from build123d import *

# Parameters (mm, degrees)
PAD043_DEPTH        = 12.5
PAD044_DEPTH        = 57
PAD046_DEPTH        = 15
CUT_PLACEMENT_ANGLE = 180


with BuildPart() as body024:
    # Sketch100 → Pad043 (new body, symmetric)
    with BuildSketch(Plane.YZ):
        Polygon((43.43318, 10), (54.734671, 10), (60, 0), (48.698509, 0), align=None)
    extrude(amount=PAD043_DEPTH, both=True)


with BuildPart() as body024_1:
    # Body024 placement: moved
    add(body024.part.moved(Location((28.5, 0, 0))))


with BuildPart() as cut:
    # Sketch099 → Pad044 (new body)
    with BuildSketch(Plane.YZ):
        Polygon((0, 0), (60, 0), (54.734671, 10), (0, 10), align=None)
    extrude(amount=PAD044_DEPTH)

    # Sketch103 (on Face1 of Pad044) → Pad046 (join)
    with BuildSketch(Plane(origin=(0, 0, 10), x_dir=(0, -1, 0), z_dir=(0, 0, 1))):
        Polygon((0, 0), (-13.5, 0), (-13.5, 5), (-5, 5), (-5, 13.5), (0, 13.5), align=None)
        Polygon((0, 57), (-13.5, 57), (-13.5, 52), (-5, 52), (-5, 43.5), (0, 43.5), align=None)
    extrude(amount=PAD046_DEPTH)

    # Cut: cut Body024
    add(body024_1.part, mode=Mode.SUBTRACT)


with BuildPart() as cut_1:
    # Cut placement: moved
    add(cut.part.moved(Location((0, 5, 0))).rotate(Axis((0, 5, 0), (0, 1, 0)), CUT_PLACEMENT_ANGLE))


solid = cut_1.part
Geometry: final body of the model. Coordinates: model frame, mm. A direction names the side the tool comes from. Round coordinates to 2 decimals unless told otherwise and drop trailing zeros. Loops run counter-clockwise (first coordinate to the right, second up) from the corner with the lowest first, then second, coordinate; pieces in that order, holes last. Notation, with made-up numbers: M 67.25,83 L 116.25,83 A20 cw 116.25,96 Z; hole C 20.25,58.25 d1. An arc over 180 degrees is marked long. Put each result on its own line as item: value. Start each with the question number.
(1) Section query D-D (y = 12). Return loops of the section in (x, z), then the cut area to 3 significant figures.
(2) Set-up query: faces 1 (the face through (-2, 18.5, -17)), 2 (the face through (-43.5, 8, -17)), 3 (the face through (-4, 10, -25)), 4 (the face through (-9, 10, -17)). Return all of +Z, -Z, +X, -X, +Y, -Y with unobstructed straight access to the full face (end or side cutting, diameter ignored); none if empty.
(3) Section query B-B (z = -13). Return loops of the section in (x, y).
(4) Material intervals for line 1 along X through (y, z) = (53.5, -9.5); line 2 along X through (y, z) = (8.5, -20.25); line 3 along Z through (x, y) = (-35, 11), sorted ascending. Write a range as [from, to].
(5) Contact query for flat-ended pins moving along their axis: pin 1 Ø4 at (x, z) = (-48.5, -20) entering from +Y; pin 2 Ø3 at (x, y) = (-39.5, 37) entering from -Z; pin 3 Ø5.5 at (x, z) = (-2, -19.5) entering from +Y. Output: stop coordinate, or through.
(6) Section query A-A (y = 57). Return loops of the section in (x, z).
(7) Draft query along X for faces 5 (the face through (-57, 28, -7)), 6 (the face through (-16, 57, -5)), 7 (the face through (-55, 18.5, -17)). Return one class per face: +X half, -X half, draft (parallel to the pull), parting line (faces both ways), or undercut.
(8) Section query C-C (x = -48). Return loops of the section in (y, z), then the cut area to 3 significant figures.
Findings below:
1. outline: M -57,-25 L -52,-25 L -52,-10 L -5,-10 L -5,-25 L 0,-25 L 0,0 L -57,0 Z
1. area: 720 mm2
2. face 1: -Z, +X, -X, +Y
2. face 2: -Z, +Y, -Y
2. face 3: -Z, +X, -X, +Y, -Y
2. face 4: -Z, +Y
3. outline: M -57,5 L -43.5,5 L -43.5,10 L -52,10 L -52,18.5 L -57,18.5 Z; M -13.5,5 L 0,5 L 0,18.5 L -5,18.5 L -5,10 L -13.5,10 Z
4. line 1: x = [-57, -41], [-16, 0]
4. line 2: x = [-57, -43.5], [-13.5, 0]
4. line 3: z = [-10, 0]
5. pin 1: stops at y = 10
5. pin 2: stops at z = -10
5. pin 3: stops at y = 18.5
6. outline: M -57,-10 L -41,-10 L -41,0 L -57,0 Z; M -16,-10 L 0,-10 L 0,0 L -16,0 Z
7. face 5: -X half
7. face 6: undercut
7. face 7: draft
8. outline: M 5,-25 L 10,-25 L 10,-10 L 59.73,-10 L 65,0 L 5,0 Z
8. area: 649 mm2
